from build123d import *

# Parameters (mm, degrees)
BOSS_EXTRUDE1_DEPTH         = 117.475
F_1_4_20_TAPPED_HOLE1_D     = 5.1054
F_1_4_20_TAPPED_HOLE1_DEPTH = 22.86
F_1_4_20_TAPPED_HOLE1_TIP   = 1.533816902
F_1_4_20_TAPPED_HOLE2_D     = 5.1054
F_1_4_20_TAPPED_HOLE2_DEPTH = 23.9014
F_1_4_20_TAPPED_HOLE2_TIP   = 1.533816902


with BuildPart() as part:
    # Sketch1 → Boss-Extrude1 (new body)
    with BuildSketch(Plane.XY):
        Polygon((-3.302, 6.35), (-6.35, 3.302), (-6.35, -47.752), (-3.302, -50.8), (3.302, -50.8), (6.35, -47.752), (6.35, 3.302), (3.302, 6.35), align=None)
    extrude(amount=BOSS_EXTRUDE1_DEPTH)

    # 1/4-20 Tapped Hole1
    with Locations(Plane.XY.offset(117.475)):
        with Locations((0, 0), (0, -44.45)):
            Hole(F_1_4_20_TAPPED_HOLE1_D / 2, depth=F_1_4_20_TAPPED_HOLE1_DEPTH)
            with Locations((0, 0, -(F_1_4_20_TAPPED_HOLE1_DEPTH + F_1_4_20_TAPPED_HOLE1_TIP / 2))):  # 118° drill point
                Cone(0, F_1_4_20_TAPPED_HOLE1_D / 2, F_1_4_20_TAPPED_HOLE1_TIP, mode=Mode.SUBTRACT)

    # 1/4-20 Tapped Hole2
    with Locations(Plane(origin=(0, 0, 0), x_dir=(-1, 0, 0), z_dir=(0, 0, -1))):
        with Locations((0, 0), (0, -44.243867412)):
            Hole(F_1_4_20_TAPPED_HOLE2_D / 2, depth=F_1_4_20_TAPPED_HOLE2_DEPTH)
            with Locations((0, 0, -(F_1_4_20_TAPPED_HOLE2_DEPTH + F_1_4_20_TAPPED_HOLE2_TIP / 2))):  # 118° drill point
                Cone(0, F_1_4_20_TAPPED_HOLE2_D / 2, F_1_4_20_TAPPED_HOLE2_TIP, mode=Mode.SUBTRACT)


solid = part.part
Here's how the part is built. I have some questions about the finished solid (model axes, mm). A direction names the side the tool comes from. Coordinates: 2 decimals unless noted, no trailing zeros. Order: outer loops, then holes, each group sorted by start corner. A loop starts at its lowest first (then second) coordinate and runs counter-clockwise, first axis right, second up. Notation, with made-up numbers: (-31, 15.25) -> (20, 15.25) arc R7 cw to (20, 27.25) -> close; hole circle Ø10 at (11.5, -4.5). An arc over 180 degrees is marked (long way). Answer in a Markdown table with one row per item.
(1) I want a section at A-A on z = 60.5. List the corners of the cut face in (x, y) for me.
Answer key:
| item | result |
|---|---|
| outline | (-6.35, -47.75) -> (-3.3, -50.8) -> (3.3, -50.8) -> (6.35, -47.75) -> (6.35, 3.3) -> (3.3, 6.35) -> (-3.3, 6.35) -> (-6.35, 3.3) -> close |
(2) I want a section at C-C on x = 5. List the corners of the cut face in (y, z) for me (3 decimals), then the cut area to 3 significant figures.
Answer key:
| item | result |
|---|---|
| outline | (-49.102, 0) -> (4.652, 0) -> (4.652, 117.475) -> (-49.102, 117.475) -> close |
| area | 6,310 mm^2 |
(3) I want a section at B-B on z = 108. List the corners of the cut face in (x, y) for me.
Answer key:
| item | result |
|---|---|
| outline | (-6.35, -47.75) -> (-3.3, -50.8) -> (3.3, -50.8) -> (6.35, -47.75) -> (6.35, 3.3) -> (3.3, 6.35) -> (-3.3, 6.35) -> (-6.35, 3.3) -> close; hole circle Ø5.11 at (0, -44.45); hole circle Ø5.11 at (0, 0) |
(4) Will these pins go through, and if not, where does the flat tip stop? pin 1 Ø3 at (x, y) = (0, -44.24) entering from +Z; pin 2 Ø1 at (x, z) = (-3.5, 53.5) entering from +Y; pin 3 Ø2 at (x, z) = (-5, 64.5) entering from -Y; pin 4 Ø3 at (x, y) = (0, 0) entering from +Z.
Answer key:
| item | result |
|---|---|
| pin 1 | z = 94.11 |
| pin 2 | y = 6.35 |
| pin 3 | y = -50.1 |
| pin 4 | z = 93.98 |
(5) Please list where these lines run through material, in increasing order: probe 1 along Y at (x, z) = (0, 13.5); probe 2 along Y at (x, z) = (0, 109); probe 3 along X at (y, z) = (0, 107.25).
Answer key:
| item | result |
|---|---|
| probe 1 | -50.8 to -46.8, -41.69 to -2.55, 2.55 to 6.35 |
| probe 2 | -50.8 to -47, -41.9 to -2.55, 2.55 to 6.35 |
| probe 3 | -6.35 to -2.55, 2.55 to 6.35 |
(6) Thinking about a two-plate mould opening in Y: for faces 4 (the face through (-0.332, -41.713, 12.118)), 5 (the face through (-2.435, 0.767, 105.885)), 6 (the face through (-4.8, -49.3, 57.9)), 7 (the face through (-6.35, -22, 58)), which applies, +Y half, -Y half, draft (parallel to the pull), parting line (faces both ways), or undercut?
Answer key:
| item | result |
|---|---|
| face 4 | undercut |
| face 5 | undercut |
| face 6 | -Y half |
| face 7 | draft |
(7) On a 3-axis mill with a long thin cutter (end or side, diameter ignored), from which of +Z, -Z, +X, -X, +Y, -Y can I reach the whole of each face in a straight line? I mean faces 1 (the face through (2.435, 0.767, 12.118)), 2 (the face through (0.33, -41.92, 105.88)), 3 (the face through (0, 6.35, 58)). Say none if no direction works.
Answer key:
| item | result |
|---|---|
| face 1 | -Z |
| face 2 | +Z |
| face 3 | +Z, -Z, +X, -X, +Y |
